Can you work these out from the model? Positions are in its coordinate system, mm. A direction names the side the tool comes from. Coordinates: 2 decimals unless noted, no trailing zeros. Loops run counter-clockwise (first coordinate to the right, second up) from the corner with the lowest first, then second, coordinate; pieces in that order, holes last.
```python
from build123d import *

# Parameters (mm, degrees)
SKETCH5_R           = 4.7625
BOSS_EXTRUDE3_DEPTH = 12.7
CHAMFER1_SIZE       = 1.190625
BOSS_EXTRUDE4_DEPTH = 6.35
SKETCH8_OUTSIDE_W   = 91.538
SKETCH8_OUTSIDE_H   = 93.748
SKETCH8_OUTSIDE_R   = 7.14375
CUT_EXTRUDE3_DEPTH  = 20.05
CUT_EXTRUDE3_TAPER  = 60


with BuildPart() as part:
    # Sketch5 → Boss-Extrude3 (new body)
    with BuildSketch(Plane(origin=(9.525, 0, 0), x_dir=(0, 0, -1), z_dir=(1, 0, 0))):
        Circle(SKETCH5_R)
    extrude(amount=-BOSS_EXTRUDE3_DEPTH)

    # Chamfer1
    chamfer1_edges = [part.edges().sort_by_distance(p)[0] for p in [
        (9.525, 0, 4.7625),
    ]]
    chamfer(chamfer1_edges, length=CHAMFER1_SIZE)



with BuildPart() as body_2:
    # Sketch6 → Boss-Extrude4 (new body)
    with BuildSketch(Plane.ZY.offset(3.175)):
        Polygon((7.14375, 4.124445986), (0, 8.248891971), (-7.14375, 4.124445986), (-7.14375, -4.124445986), (0, -8.248891971), (7.14375, -4.124445986), align=None)
    extrude(amount=BOSS_EXTRUDE4_DEPTH)

    # Sketch8 outside → Cut-Extrude3 (cut, through all)
    with BuildSketch(Plane.ZY.offset(9.525)):
        Rectangle(SKETCH8_OUTSIDE_W, SKETCH8_OUTSIDE_H)
        Circle(SKETCH8_OUTSIDE_R, mode=Mode.SUBTRACT)
    extrude(amount=-CUT_EXTRUDE3_DEPTH, taper=CUT_EXTRUDE3_TAPER, mode=Mode.SUBTRACT)


with BuildPart() as part_1:
    add(part.part)

    add(body_2.part)  # Revolve7 merges body 2
    # Sketch13 → Revolve7 (revolve)
    with BuildSketch(Plane.XY):
        Polygon((-3.429, 0), (5.084670523, 0), (-3.175, 4.768723), (-3.429, 4.768723), align=None)
    revolve(axis=Axis((-3.429, 0, 0), (1, 0, 0)))


solid = part_1.part
```
Item 1: I need wall thicknesses on line 1 along X through (y, z) = (-6.25, -0.5) (3 decimals); line 2 along Z through (x, y) = (5.25, 0); line 3 along Y through (x, z) = (-8.5, -5.5). Which ranges of each line are inside material? Lowest first, please.
Results are:
line 1: x = -9.525 to -3.175
line 2: z = -4.76 to 4.76
line 3: y = -5.07 to 5.07
Item 2: Suppose I cut it at A-A, the plane x = -2.75. Please give me the cut outline in (y, z) (1 decimal), plus the area to 3 significant figures.
Results are:
outline: circle Ø9.5 at (0, 0)
area: 71.3 mm2
Item 3: On a 3-axis mill with a long thin cutter (end or side, diameter ignored), from which of +Z, -Z, +X, -X, +Y, -Y can I reach the whole of each face in a straight line? I mean faces 1 (the face through (-3.175, -4, -3)), 2 (the face through (-6.31, 6.16, 3.62)). Say none if no direction works.
Results are:
face 1: +X
face 2: +Z, +X, -X, +Y
Item 4: I'm going to push flat-ended pins straight in: P1, Ø4, axis at x = 0.5, y = -5, coming from the +Z side; P2, Ø6, axis at x = 4, z = -3.5, coming from the -Y side; P3, Ø1, axis at x = -3, z = 2, coming from the +Y side. Where does each tip first touch, or does it pass through?
Results are:
P1: stops at z = 3.7
P2: stops at y = -4.74
P3: stops at y = 7.36
